Can you work these out from the model? Positions are in its coordinate system, mm. A direction names the side the tool comes from. Round coordinates to 2 decimals unless told otherwise and drop trailing zeros. Loops run counter-clockwise (first coordinate to the right, second up) from the corner with the lowest first, then second, coordinate; pieces in that order, holes last. Notation, with made-up numbers: (72.25, 15) -> (80.25, 15) arc R35 cw to (80.25, 50) -> close; hole circle Ø5 at (-17.5, 40). An arc over 180 degrees is marked (long way). Write item = value, one per line.
from build123d import *

# Parameters (mm, degrees)
F0_R     = 35.128120954
F0_R_2   = 29.9814765583
F1_DEPTH = 34
F3_DEPTH = 56.7
F4_DEPTH = 15
F5_DEPTH = 15
F6_DEPTH = 15
F7_DEPTH = 15


# Not quite as in the source:
# - a feature names something its author has since deleted; it is built from what else it names


with BuildPart() as f1:
    # F0 (on Top) → F1 (new body)
    with BuildSketch(Plane.XY):
        Circle(F0_R)
        Circle(F0_R_2, mode=Mode.SUBTRACT)
    extrude(amount=F1_DEPTH)

    # F2 (on Top) → F3 (cut)
    with BuildSketch(Plane.XY):
        Polygon((0, 50.666205585), (0, 0), (-44.6641780436, 0), (-44.6641780436, -44.4084256887), (0, -44.4084256887), (0, -49.6323108673), (44.1417917609, -49.6323108673), (44.1417917609, 0), (47.7985069156, 0), (47.7985069156, 50.666205585), align=None)
    extrude(amount=F3_DEPTH, mode=Mode.SUBTRACT)

    # F4 (add): a face of the model
    f4_faces = [f1.faces().sort_by_distance(p)[0] for p in [
        (0, 32.5547987561, 17),
    ]]
    extrude(f4_faces, amount=F4_DEPTH)

    # F5 (add): a face of the model
    f5_faces = [f1.faces().sort_by_distance(p)[0] for p in [
        (-32.5547987561, 0, 17),
    ]]
    extrude(f5_faces, amount=F5_DEPTH)

    # F6 (add): a face of the model
    f6_faces = [f1.faces().sort_by_distance(p)[0] for p in [
        (-32.5547987561, -15, 17),
    ]]
    extrude(f6_faces, amount=F6_DEPTH)

    # F7 (add): a face of the model
    f7_faces = [f1.faces().sort_by_distance(p)[0] for p in [
        (15, 32.5547987561, 17),
    ]]
    extrude(f7_faces, amount=F7_DEPTH)


solid = f1.part
1. Suppose I cut it at B-B, the plane y = -17. List the corners of the cut face in (x, z) for me, and give its area (3 significant figures).
Entries:
outline = (-35.13, 0) -> (-29.98, 0) -> (-29.98, 34) -> (-35.13, 34) -> close
area = 175 mm²
2. Suppose I cut it at A-A, the plane z = 7.5. List the corners of the cut face in (x, y) for me.
Entries:
outline = (-35.13, -30) -> (-29.98, -30) -> (-29.98, 0) arc R29.98 cw to (0, 29.98) -> (30, 29.98) -> (30, 35.13) -> (0, 35.13) arc R35.13 ccw to (-35.13, 0) -> close
3. For faces 1 (the flat face through (-29.981, -15, 17)), 2 (the flat face through (-35.128, -15, 17)), which set-ups out of +Z, -Z, +X, -X, +Y, -Y let a thin tool reach every point of the face, with its end or its side?
Entries:
face_1 = +Z, -Z, +X, -Y
face_2 = +Z, -Z, -X, +Y, -Y
4. Suppose I cut it at C-C, the plane x = 2.5. List the corners of the cut face in (y, z) for me.
Entries:
outline = (29.98, 0) -> (35.13, 0) -> (35.13, 34) -> (29.98, 34) -> close
5. I need wall thicknesses on line 1 (X direction, y = -23, z = 4); line 2 (Y direction, x = 2, z = 20); line 3 (X direction, y = 27, z = 27). Which ranges of each line are inside material? Lowest first, please. Write a range as [from, to].
Entries:
line_1 = [-35.13, -29.98]
line_2 = [29.98, 35.13]
line_3 = [-22.47, -13.03]
6. I'm going to push flat-ended pins straight in: pin 1 (15 mm diameter, centred on x = 14.5, z = 17, fed in from -Y); pin 2 (3 mm diameter, centred on x = -27, y = -21, fed in from -Z); pin 3 (8 mm diameter, centred on y = -10, z = 28, fed in from +X); pin 4 (12 mm diameter, centred on x = -16, z = 22, fed in from +Y). Where does each tip first touch, or does it pass through?
Entries:
pin_1 = 29.98
pin_2 = through
pin_3 = -29.98
pin_4 = 33.67
7. We'd pull the mould along Y, two halves only. Please class faces 3 (the flat face through (-22, 22, 0)), 4 (the flat face through (15, 35.128, 17)), 5 (the flat face through (15, 29.981, 17)): released by +Y, released by -Y, zero draft, split by the parting line, or undercut.
Entries:
face_3 = zero draft
face_4 = released by +Y
face_5 = released by -Y
